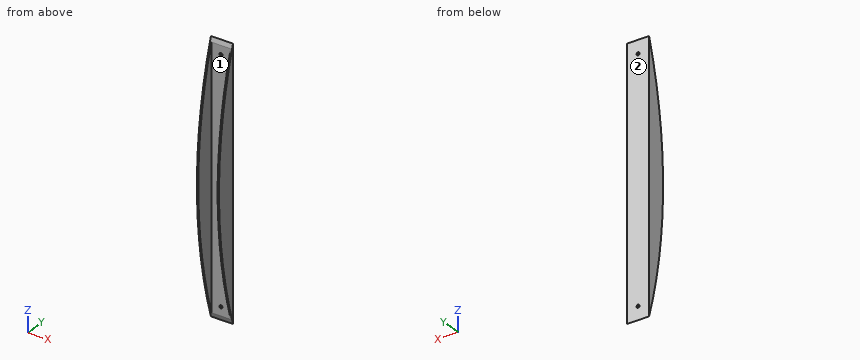
from build123d import *

# Parameters (mm, degrees)
F0_W     = 25.4
F0_H     = 300
F1_DEPTH = 25.4
F2_W     = 22.225
F2_H     = 22.225
F3_DEPTH = 300
F5_DEPTH = 25.4
F6_R     = 1.75
F7_DEPTH = 25


with BuildPart() as f1:
    # F0 (on Right) → F1 (new body)
    with BuildSketch(Plane.YZ):
        with Locations((12.7, 150)):
            Rectangle(F0_W, F0_H)
    extrude(amount=F1_DEPTH)

    # F2 (on face) → F3 (cut)
    with BuildSketch(Plane.XY.offset(300)):
        with Locations((12.7, 12.7)):
            Rectangle(F2_W, F2_H)
    extrude(amount=-F3_DEPTH, mode=Mode.SUBTRACT)

    # F4 (on face) → F5 (cut)
    with BuildSketch(Plane.YZ.offset(25.4)):
        with BuildLine():
            ThreePointArc((25.4, 0), (2.775952, 150), (25.4, 300))
            Line((25.4, 300), (0, 300))
            Line((0, 300), (0, 0))
            Line((0, 0), (25.4, 0))
        make_face()
    extrude(amount=-F5_DEPTH, mode=Mode.SUBTRACT)

    # F6 (on face) → F7 (cut)
    with BuildSketch(Plane(origin=(0, 25.4, 0), x_dir=(-1, 0, 0), z_dir=(0, 1, 0))):
        with Locations((-12.7, 285)):
            Circle(F6_R)
        with Locations((-12.7, 15)):
            Circle(F6_R)
    extrude(amount=-F7_DEPTH, mode=Mode.SUBTRACT)


solid = f1.part
Geometry check sheet. Reference: the model listing, model coordinates, mm. Face numbers are marked on the shaded views. Give positions to 0.01 mm unless a question says otherwise; leave off trailing zeros. Write each loop counter-clockwise with the first axis right and the second up, starting at its lowest first coordinate (ties: lowest second). Pieces come first, ordered by that corner, then holes. Notation, with made-up numbers: M 74.25,16 L 132.25,16 A17 cw 132.25,20 Z; hole C 43,35 d6. An arc over 180 degrees is marked long. One line per question, with ' | ' between items.
1. Cross-section at B-B (z = 188.5). Enter the section's corners in (x, y), plus the area to 3 significant figures.
Ans:
outline: M 0,4.24 L 1.59,4.24 L 1.59,23.81 L 23.81,23.81 L 23.81,4.24 L 25.4,4.24 L 25.4,25.4 L 0,25.4 Z | area: 102 mm2
2. Cross-section at D-D (y = 21.25). Enter the section's corners in (x, z).
Ans:
outline: M 0,14.17 L 1.59,14.17 L 1.59,285.83 L 0,285.83 Z; M 23.81,14.17 L 25.4,14.17 L 25.4,285.83 L 23.81,285.83 Z
3. Cross-section at C-C (x = 17.5). Enter the section's corners in (y, z).
Ans:
outline: M 23.81,5.24 A508.57 ccw 25.4,0 L 25.4,300 A508.57 ccw 23.81,294.76 Z
4. Gauge pin test, flat ends, axial feed: pin 1 (1.5 mm diameter, centred on x = 18.5, y = 21.5, fed in from -Z); pin 2 (3 mm diameter, centred on x = 14, z = 248, fed in from -Y); pin 3 (6 mm diameter, centred on y = 22.5, z = 40.5, fed in from -X). Record the tip position at first contact, or that the pin passes through.
Ans:
pin 1: through | pin 2: y = 23.81 | pin 3: x = 0
5. Mould release check, pull along X, two halves, no side actions. Record for the marked faces 1 and 2: released by +X, released by -X, zero draft, split by the parting line, or undercut.
Ans:
face 1: undercut | face 2: zero draft
6. Scan lines: line 1 along X through (y, z) = (23.25, 203); line 2 along X through (y, z) = (24.95, 285); line 3 along Y through (x, z) = (7.5, 213). Record each from-to range of solid material in increasing order. Write a range as from..to.
Ans:
line 1: 0..1.59, 23.81..25.4 | line 2: 0..10.95, 14.45..25.4 | line 3: 23.81..25.4
